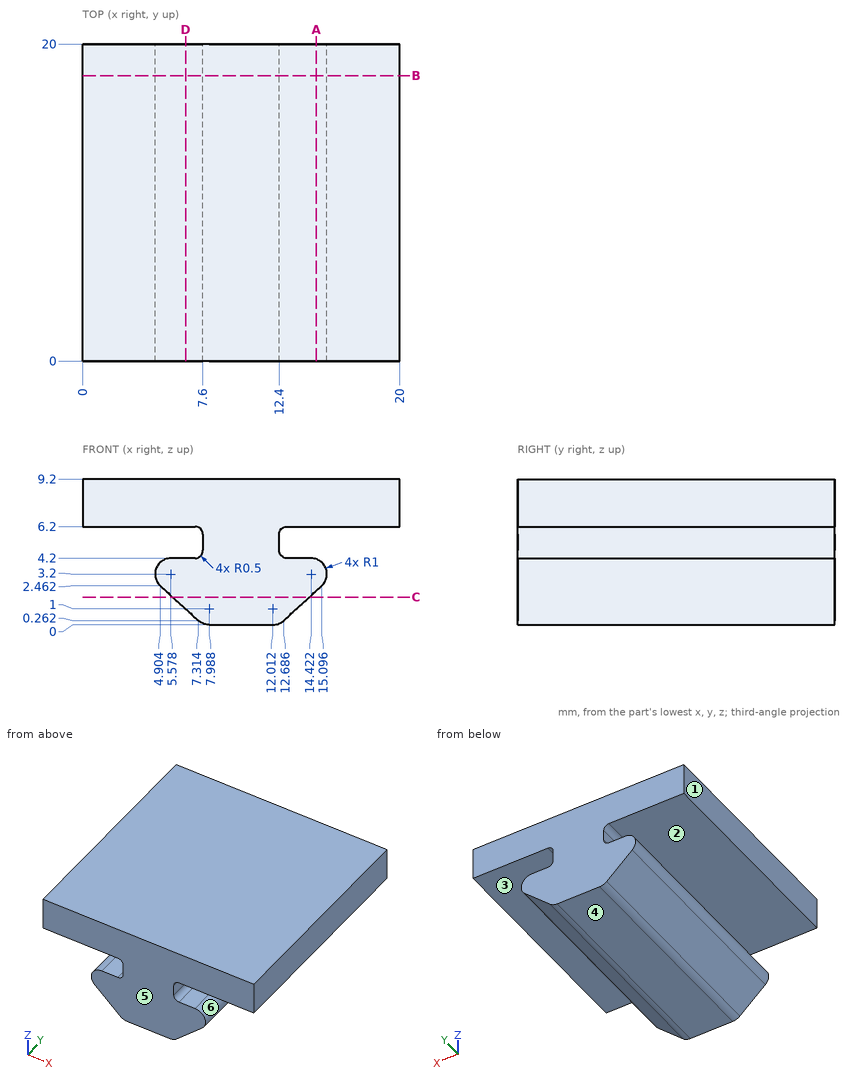
Part print with two shaded views. Sizes in mm from the minimum x, y, z corner. A direction names the side the tool comes from. Give positions to 0.01 mm unless a question says otherwise; leave off trailing zeros. Order: outer loops, then holes, each group sorted by start corner. A loop starts at its lowest first (then second) coordinate and runs counter-clockwise, first axis right, second up.
(1) Saw through at B-B, the plane y = 18. Give the cut face in (x, z) (1 decimal).
(2) Saw through at C-C, the plane z = 1.75. Give the cut face in (x, y).
(3) Drill centre lines: L1, parallel to X at y = 14.75, z = 5.75; L2, parallel to Z at x = 14.5, y = 14 (1 decimal); L3, parallel to Z at x = 17, y = 5.5. Where is each one in solid material? Low to high.
(4) Mould opens along Z. For the marked faces 4, 5 and 6 say: released by +Z, released by -Z, zero draft, split by the parting line, or undercut.
(5) Saw through at A-A, the plane x = 14.75. Give the cut face in (y, z) (1 decimal).
(6) Flat gauge pins, fed straight in: pin 1 (1 mm diameter, centred on y = 17.5, z = 5.5, fed in from +X); pin 2 (0.8 mm diameter, centred on y = 9.5, z = 5, fed in from -X); pin 3 (2 mm diameter, centred on x = 2.5, y = 13, fed in from -Z); pin 4 (3 mm diameter, centred on x = 17, z = 2.5, fed in from +Y). Where does each tip first touch, or does it go through?
(7) Tool access for the marked faces 1, 2 and 3: list every direction of +Z, -Z, +X, -X, +Y, -Y with a clear straight run to the whole face (end or side of a thin tool).
(8) Saw through at D-D, the plane x = 6.5. Give the cut face in (y, z) (1 decimal), then the cut area to 3 significant figures.
Results found:
1. outline: (0, 6.2) - (7.1, 6.2) arc R0.5 cw to (7.6, 5.7) - (7.6, 4.7) arc R0.5 cw to (7.1, 4.2) - (5.6, 4.2) arc R1 ccw to (4.9, 2.5) - (7.3, 0.3) arc R1 ccw to (8, 0) - (12, 0) arc R1 ccw to (12.7, 0.3) - (15.1, 2.5) arc R1 ccw to (14.4, 4.2) - (12.9, 4.2) arc R0.5 cw to (12.4, 4.7) - (12.4, 5.7) arc R0.5 cw to (12.9, 6.2) - (20, 6.2) - (20, 9.2) - (0, 9.2) - close
2. outline: (5.68, 0) - (14.32, 0) - (14.32, 20) - (5.68, 20) - close
3. L1: x = 7.6 to 12.4
3. L2: z = 1.9 to 4.2, 6.2 to 9.2
3. L3: z = 6.2 to 9.2
4. face 4: released by -Z
4. face 5: zero draft
4. face 6: undercut
5. outline: (0, 2.1) - (20, 2.1) - (20, 4.1) - (0, 4.1) - close; (0, 6.2) - (20, 6.2) - (20, 9.2) - (0, 9.2) - close
6. pin 1: stops at x = 12.5
6. pin 2: stops at x = 7.59
6. pin 3: stops at z = 6.2
6. pin 4: passes through
7. face 1: +Z, -Z, -X, +Y, -Y
7. face 2: -X, +Y, -Y
7. face 3: +X, +Y, -Y
8. outline: (0, 1) - (20, 1) - (20, 4.2) - (0, 4.2) - close; (0, 6.2) - (20, 6.2) - (20, 9.2) - (0, 9.2) - close
8. area: 124 mm2
